Source: three-view drawing plus pictorial views. Frame: mm from the lowest corner of the part. Give positions to 0.01 mm unless a question says otherwise; leave off trailing zeros. Loops run counter-clockwise (first coordinate to the right, second up) from the corner with the lowest first, then second, coordinate; pieces in that order, holes last. Notation, with made-up numbers: (-1, 37.5) - (43, 37.5) arc R20 ccw to (43, 55.5) - close; hole circle Ø3 at (72.5, -3). An arc over 180 degrees is marked (long way). Answer as a JSON object with one key per item and string values.
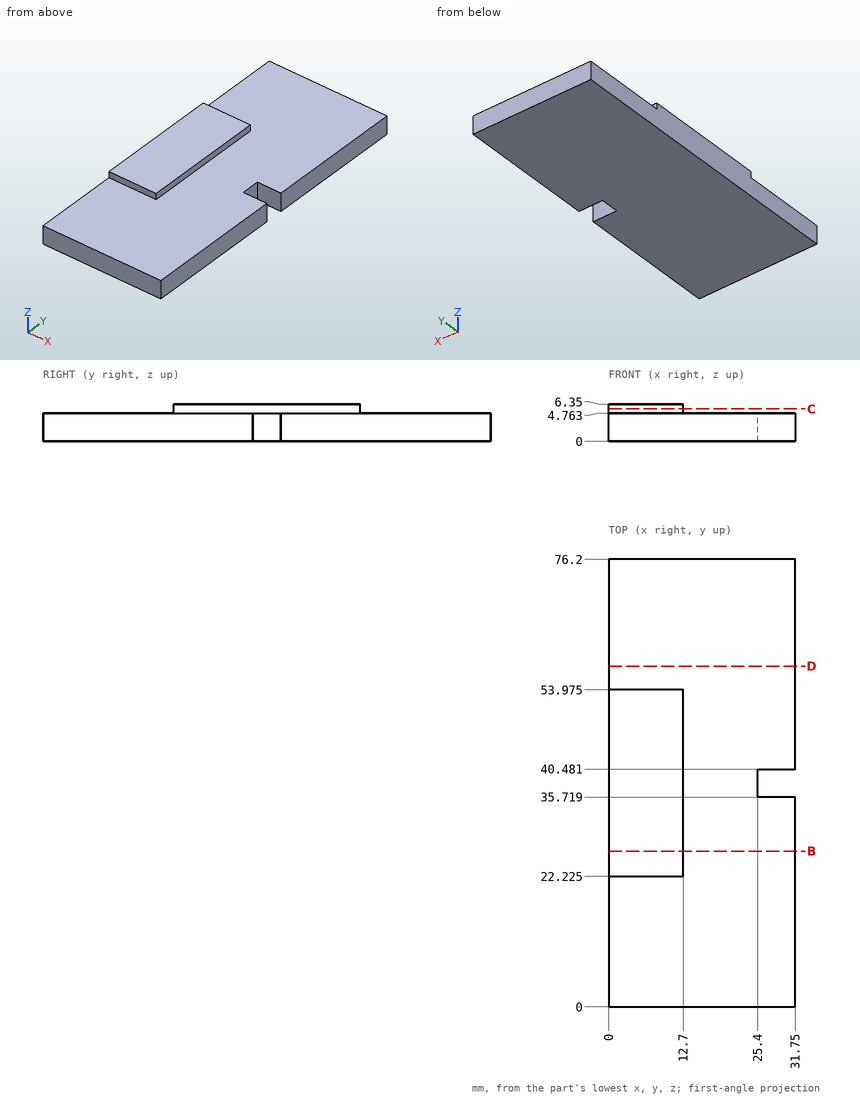
Item 1: Cut plane C-C (z = 5.5). Return loops of the section in (x, y) (1 decimal).
Geometry check:
{"outline": "(0, 22.2) - (12.7, 22.2) - (12.7, 54) - (0, 54) - close"}
Item 2: Material intervals for line 1 (Y direction, x = 28, z = 4.5); line 2 (Z direction, x = 20.5, y = 48.5); line 3 (X direction, y = 30, z = 6), sorted ascending. Write a range as [from, to].
Geometry check:
{"line 1": "y = [0, 35.72], [40.48, 76.2]", "line 2": "z = [0, 4.76]", "line 3": "x = [0, 12.7]"}
Item 3: Cut plane D-D (y = 58). Return loops of the section in (x, z).
Geometry check:
{"outline": "(0, 0) - (31.75, 0) - (31.75, 4.76) - (0, 4.76) - close"}
Item 4: Contact query for flat-ended pins moving along their axis: P1, Ø1.3, axis at y = 35, z = 6, coming from the +X side; P2, Ø1.7, axis at x = 9.5, z = 6, coming from the +Y side (1 decimal); P3, Ø8, axis at x = 6.5, y = 68, coming from the +Z side. Output: stop coordinate, or through.
Geometry check:
{"P1": "stops at x = 12.7", "P2": "stops at y = 54", "P3": "stops at z = 4.76"}
Item 5: Cut plane B-B (y = 26.5). Return loops of the section in (x, z).
Geometry check:
{"outline": "(0, 0) - (31.75, 0) - (31.75, 4.76) - (12.7, 4.76) - (12.7, 6.35) - (0, 6.35) - close"}
